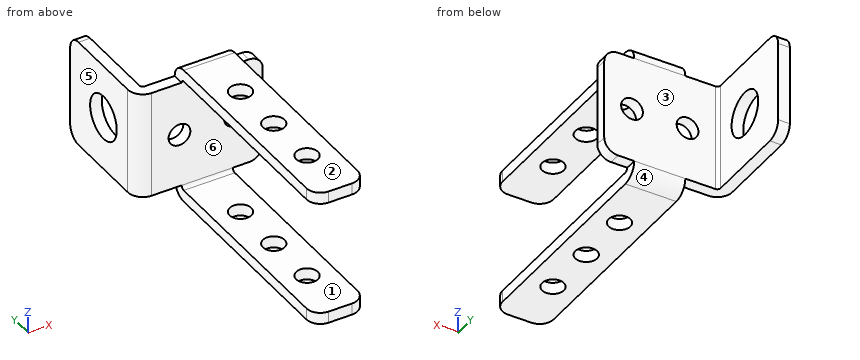
```python
from build123d import *

# Parameters (mm, degrees)
BASE_FLANGE1_START       = -12.7
BASE_FLANGE1_DEPTH       = 25.4
EDGE_FLANGE1_DEPTH       = 24.638
SKETCH9_R                = 5.08
CUT_EXTRUDE1_DEPTH       = 86.568694538
CUT_EXTRUDE2_START       = -12.7
CUT_EXTRUDE2_DEPTH       = 6.858
CUT_EXTRUDE2_START_2     = 5.842
CUT_EXTRUDE2_2_DEPTH     = 6.858
CUT_EXTRUDE2_START_3     = -28.829
CUT_EXTRUDE2_3_OUTLINE_R = 2.4892
CUT_EXTRUDE2_3_DEPTH     = 31.496
CUT_EXTRUDE3_REACH       = 64.849
SKETCH11_R               = 2.4892
FILLET1_R                = 3.175


with BuildPart() as part:
    # Base-Flange1: read off the stored shape, not the designer's step
    # Base-Flange1 outline → Base-Flange1 (new body)
    with BuildSketch(Plane(origin=(0, 0, 0), x_dir=(0, 0, -1), z_dir=(1, 0, 0)).offset(BASE_FLANGE1_START)):
        with BuildLine():
            Line((26.162, 50.038), (26.162, 0))
            Line((26.162, 0), (28.829, 0))
            Line((28.829, 0), (28.829, 50.038))
            ThreePointArc((28.829, 50.038), (27.824669153, 52.462669153), (25.4, 53.467))
            Line((25.4, 53.467), (0.762, 53.467))
            ThreePointArc((0.762, 53.467), (-1.662669153, 52.462669153), (-2.667, 50.038))
            Line((-2.667, 50.038), (-2.667, 0))
            Line((-2.667, 0), (0, 0))
            Line((0, 0), (0, 50.038))
            ThreePointArc((0, 50.038), (0.223184633, 50.576815367), (0.762, 50.8))
            Line((0.762, 50.8), (25.4, 50.8))
            ThreePointArc((25.4, 50.8), (25.938815367, 50.576815367), (26.162, 50.038))
        make_face()
    extrude(amount=BASE_FLANGE1_DEPTH)

    # Edge-Flange1: sheet metal written as solids
    # Edge-Flange1 section (on a plane across the edge) → Edge-Flange1 (add)
    with BuildSketch(Plane(origin=(-13.462, 53.467, -25.4), x_dir=(1, 0, 0), z_dir=(0, 0, 1))):
        with BuildLine():
            Line((-2.667, 0.762), (-2.667, 22.733))
            Line((-2.667, 22.733), (0, 22.733))
            Line((0, 22.733), (0, 0.762))
            ThreePointArc((0, 0.762), (0.223184633, 0.223184633), (0.762, 0))
            Line((0.762, 0), (0.762, -2.667))
            ThreePointArc((0.762, -2.667), (-1.662669153, -1.662669153), (-2.667, 0.762))
        make_face()
    extrude(amount=EDGE_FLANGE1_DEPTH)

    # Sketch9 → Cut-Extrude1 (cut, through all)
    with BuildSketch(Plane(origin=(-13.462, 0, 0), x_dir=(0, 0, -1), z_dir=(1, 0, 0))):
        with Locations(Location((13.081, 63.5, 0), (0, 0, 90))):
            Circle(SKETCH9_R)
    extrude(amount=-CUT_EXTRUDE1_DEPTH, mode=Mode.SUBTRACT)

    # Cut-Extrude2: read off the stored shape, not the designer's step
    # Cut-Extrude2 outline → Cut-Extrude2 (cut)
    with BuildSketch(Plane.YZ.offset(CUT_EXTRUDE2_START)):
        with BuildLine():
            Line((53.467, -25.4), (50.8, -25.4))
            ThreePointArc((50.8, -25.4), (50.576815367, -25.938815367), (50.038, -26.162))
            Line((50.038, -26.162), (0, -26.162))
            Line((0, -26.162), (0, -28.829))
            Line((0, -28.829), (50.038, -28.829))
            ThreePointArc((50.038, -28.829), (52.462669153, -27.824669153), (53.467, -25.4))
        make_face()
        with BuildLine():
            ThreePointArc((50.038, 0), (50.576815367, -0.223184633), (50.8, -0.762))
            Line((50.8, -0.762), (53.467, -0.762))
            ThreePointArc((53.467, -0.762), (52.462669153, 1.662669153), (50.038, 2.667))
            Line((50.038, 2.667), (0, 2.667))
            Line((0, 2.667), (0, 0))
            Line((0, 0), (50.038, 0))
        make_face()
    extrude(amount=CUT_EXTRUDE2_DEPTH, mode=Mode.SUBTRACT)

    # Cut-Extrude2 2 outline → Cut-Extrude2 2 (cut)
    with BuildSketch(Plane.YZ.offset(CUT_EXTRUDE2_START_2)):
        with BuildLine():
            Line((53.467, -25.4), (50.8, -25.4))
            ThreePointArc((50.8, -25.4), (50.576815367, -25.938815367), (50.038, -26.162))
            Line((50.038, -26.162), (0, -26.162))
            Line((0, -26.162), (0, -28.829))
            Line((0, -28.829), (50.038, -28.829))
            ThreePointArc((50.038, -28.829), (52.462669153, -27.824669153), (53.467, -25.4))
        make_face()
        with BuildLine():
            ThreePointArc((50.038, 0), (50.576815367, -0.223184633), (50.8, -0.762))
            Line((50.8, -0.762), (53.467, -0.762))
            ThreePointArc((53.467, -0.762), (52.462669153, 1.662669153), (50.038, 2.667))
            Line((50.038, 2.667), (0, 2.667))
            Line((0, 2.667), (0, 0))
            Line((0, 0), (50.038, 0))
        make_face()
    extrude(amount=CUT_EXTRUDE2_2_DEPTH, mode=Mode.SUBTRACT)

    # Cut-Extrude2 3 outline → Cut-Extrude2 3 (cut)
    with BuildSketch(Plane.XY.offset(CUT_EXTRUDE2_START_3)):
        with Locations((0, 12.7)):
            Circle(CUT_EXTRUDE2_3_OUTLINE_R)
        with Locations((0, 38.1)):
            Circle(CUT_EXTRUDE2_3_OUTLINE_R)
        with Locations((0, 25.4)):
            Circle(CUT_EXTRUDE2_3_OUTLINE_R)
    extrude(amount=CUT_EXTRUDE2_3_DEPTH, mode=Mode.SUBTRACT)

    # Sketch11 → Cut-Extrude3 (cut, up to next)
    with BuildSketch(Plane(origin=(0, 53.467, 0), x_dir=(1, 0, 0), z_dir=(0, 1, 0)), mode=Mode.PRIVATE) as cut_extrude3_sk1:
        with Locations(Location((-6.35, 13.081, 0), (0, 0, 270))):
            Circle(SKETCH11_R)
    cut_extrude3_tool1 = extrude(cut_extrude3_sk1.sketch, amount=-CUT_EXTRUDE3_REACH, mode=Mode.PRIVATE) & part.part
    # Sketch11 → Cut-Extrude3 (cut, up to next)
    with BuildSketch(Plane(origin=(0, 53.467, 0), x_dir=(1, 0, 0), z_dir=(0, 1, 0)), mode=Mode.PRIVATE) as cut_extrude3_sk2:
        with Locations(Location((6.35, 13.081, 0), (0, 0, 270))):
            Circle(SKETCH11_R)
    cut_extrude3_tool2 = extrude(cut_extrude3_sk2.sketch, amount=-CUT_EXTRUDE3_REACH, mode=Mode.PRIVATE) & part.part
    add(cut_extrude3_tool1.solids().sort_by_distance((-6.35, 53.467, -13.081))[0], mode=Mode.SUBTRACT)
    add(cut_extrude3_tool2.solids().sort_by_distance((6.35, 53.467, -13.081))[0], mode=Mode.SUBTRACT)

    # Fillet1
    fillet1_edges = [part.edges().sort_by_distance(p)[0] for p in [
        (5.842, 0, 1.3335),
        (-5.842, 0, 1.3335),
        (5.842, 0, -27.4955),
        (-5.842, 0, -27.4955),
        (12.7, 52.1335, -25.4),
        (12.7, 52.1335, -0.762),
        (-14.7955, 76.2, -25.4),
        (-14.7955, 76.2, -0.762),
    ]]
    fillet(fillet1_edges, radius=FILLET1_R)


solid = part.part
```
Model file for the job. Use its own axes, mm. Face numbers are marked on the shaded views. A direction names the side the tool comes from. Coordinates: 2 decimals unless noted, no trailing zeros. Order: outer loops, then holes, each group sorted by start corner. A loop starts at its lowest first (then second) coordinate and runs counter-clockwise, first axis right, second up. Notation, with made-up numbers: (-14.5, -24.5) -> (18.5, -24.5) arc R18 ccw to (18.5, -5.5) -> close; hole circle Ø6 at (45, 56). An arc over 180 degrees is marked (long way). Answer as a JSON object with one key per item and string values. Group by question number.
1) Cut at C-C, the plane x = 0. Count the separate pieces of the cut face and the enclosed holes in it, then the cut area to 3 significant figures.
2) Cut at A-A, the plane y = 48. Write the cut outline in (x, z).
3) Cut at B-B, the plane y = 12.7. Write the cut outline in (x, z).
4) Which spindle directions (+Z, -Z, +X, -X, +Y, -Y) get a long thin tool onto all of the face, cutting with end or side? Do the marked faces 1, 2 and 3. Say none if no direction does.
5) Drill centre lines: L1, parallel to X at y = 25.4, z = -26.9; L2, parallel to Z at x = 5.25, y = 26.5; L3, parallel to Y at x = 0, z = -28.1. Where is each one in solid material? Low to high.
6) Flat gauge pins, fed straight in: pin 1 (1.7 mm diameter, centred on y = 32, z = -27.5, fed in from -X); pin 2 (1 mm diameter, centred on y = 39.5, z = -27.5, fed in from +X); pin 3 (11.5 mm diameter, centred on x = -12.5, y = 67.5, fed in from +Z); pin 4 (5 mm diameter, centred on x = -8.5, y = 58, fed in from -Z). Where does each tip first touch, or does it go through?
7) Cut at D-D, the plane z = -14.5. Write the cut outline in (x, y).
8) Pull direction Z, two halves, no side cores. Call the marked faces 4, 5 and 6: +Z half, -Z half, draft (parallel to the pull), parting line (faces both ways), or undercut.
Check values:
{
 "1": {"separate pieces": "7", "enclosed holes": "0", "area": "271 mm²"},
 "2": {"outline": "(-5.84, -28.83) -> (5.84, -28.83) -> (5.84, -26.16) -> (-5.84, -26.16) -> close; (-5.84, 0) -> (5.84, 0) -> (5.84, 2.67) -> (-5.84, 2.67) -> close"},
 "3": {"outline": "(-5.84, -28.83) -> (-2.49, -28.83) -> (-2.49, -26.16) -> (-5.84, -26.16) -> close; (-5.84, 0) -> (-2.49, 0) -> (-2.49, 2.67) -> (-5.84, 2.67) -> close; (2.49, -28.83) -> (5.84, -28.83) -> (5.84, -26.16) -> (2.49, -26.16) -> close; (2.49, 0) -> (5.84, 0) -> (5.84, 2.67) -> (2.49, 2.67) -> close"},
 "4": {"face 1": "+X, -X, -Y", "face 2": "+Z, +X, -X, +Y, -Y", "face 3": "+Z, -Z, +X, +Y"},
 "5": {"L1": "x = -5.84 to -2.49, 2.49 to 5.84", "L2": "z = -28.83 to -26.16, 0 to 2.67", "L3": "y = 0 to 10.21, 15.19 to 22.91, 27.89 to 35.61, 40.59 to 52.15"},
 "6": {"pin 1": "stops at x = -5.84", "pin 2": "stops at x = 5.84", "pin 3": "stops at z = -0.76", "pin 4": "passes through"},
 "7": {"outline": "(-16.13, 54.23) arc R3.43 ccw to (-12.7, 50.8) -> (-8.4, 50.8) -> (-8.4, 53.47) -> (-12.7, 53.47) arc R0.76 cw to (-13.46, 54.23) -> (-13.46, 58.62) -> (-16.13, 58.62) -> close; (-16.13, 68.38) -> (-13.46, 68.38) -> (-13.46, 76.2) -> (-16.13, 76.2) -> close; (-4.3, 50.8) -> (4.3, 50.8) -> (4.3, 53.47) -> (-4.3, 53.47) -> close; (8.4, 50.8) -> (12.7, 50.8) -> (12.7, 53.47) -> (8.4, 53.47) -> close"},
 "8": {"face 4": "-Z half", "face 5": "draft", "face 6": "undercut"}
}
